For this review, use the dimensioned drawing (mm, ordinates from the lowest corner) and the shaded views. A direction names the side the tool comes from. Coordinates: 2 decimals unless noted, no trailing zeros. Write each loop counter-clockwise with the first axis right and the second up, starting at its lowest first coordinate (ties: lowest second). Pieces come first, ordered by that corner, then holes. Notation, with made-up numbers: M 84,12 L 143,12 A7 ccw 143,25 Z; hole C 72,89.25 d6. An arc over 180 degrees is marked long. Return JSON: item names as keys, results as strings. Group by question number.
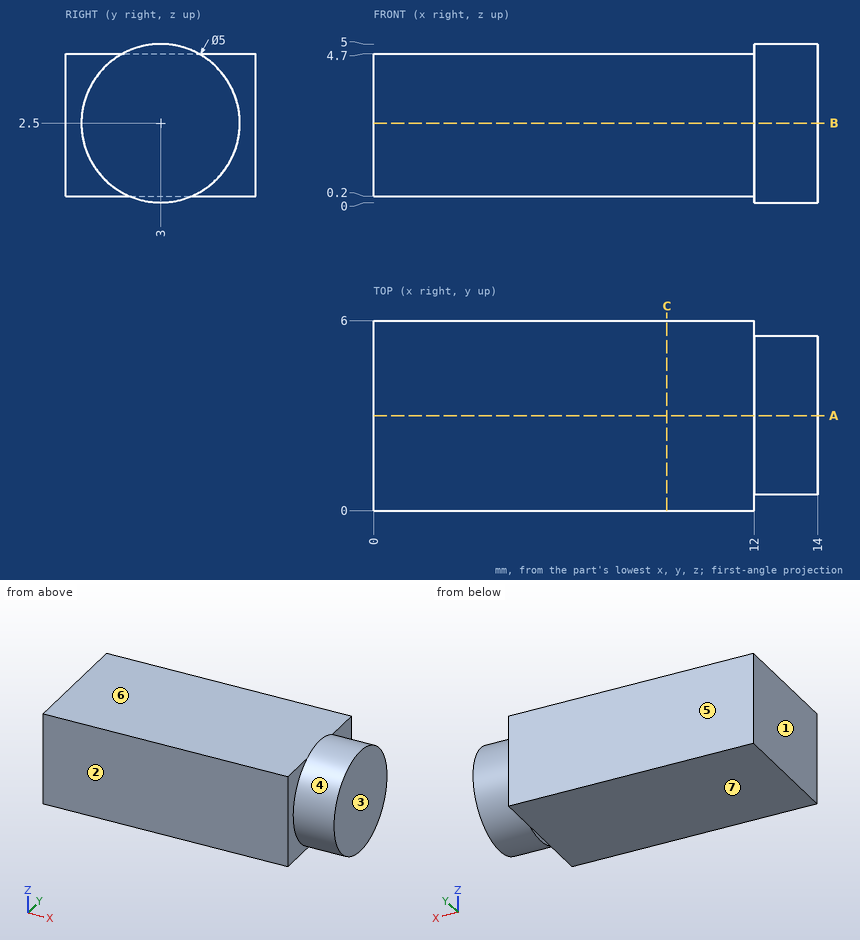
Item 1: Add section B-B (z = 2.5). Write out the cut boundary in (x, y).
Item 2: For line 1 (Z direction, x = 4.5, y = 2.3); line 2 (X direction, y = 5.5, z = 4.3); line 3 (Z direction, x = 13.5, y = 4.2), list the stretches that pass through material, from the lowest coordinate up.
Item 3: Machinability: for the marked faces 4, 5, 6 and 7, which of the approach directions +Z, -Z, +X, -X, +Y, -Y give a long, thin tool a straight path to every point of the face, cutting with its end or side? Answer none if there is none.
Item 4: For pin 1 (3 mm diameter, centred on x = 10, y = 5, fed in from -Z); pin 2 (2 mm diameter, centred on x = 10, y = 1, fed in from +Z), all flat-tipped, find the tip position at first contact; note any pin that passes through.
Item 5: The part is to be moulded in two halves that separate along X. For the marked faces 1, 2 and 3, say which applies: pulls with the +X half, pulls with the -X half, needs draft (parallel to the pull), parting line crosses it, or undercut.
Item 6: Add section A-A (y = 3). Write out the cut boundary in (x, z).
Item 7: Add section C-C (x = 9.25). Write out the cut boundary in (y, z), plus the area to 3 significant figures.
Geometry check:
{
 "1": {"outline": "M 0,0 L 12,0 L 12,0.5 L 14,0.5 L 14,5.5 L 12,5.5 L 12,6 L 0,6 Z"},
 "2": {"line 1": "0.2 to 4.7", "line 2": "0 to 12", "line 3": "0.31 to 4.69"},
 "3": {"face 4": "+X", "face 5": "+Z, -Z, +X, -X, +Y", "face 6": "+Z, -X, +Y, -Y", "face 7": "-Z, -X, +Y, -Y"},
 "4": {"pin 1": "z = 0.2", "pin 2": "z = 4.7"},
 "5": {"face 1": "pulls with the -X half", "face 2": "needs draft", "face 3": "pulls with the +X half"},
 "6": {"outline": "M 0,0.2 L 12,0.2 L 12,0 L 14,0 L 14,5 L 12,5 L 12,4.7 L 0,4.7 Z"},
 "7": {"outline": "M 0,0.2 L 6,0.2 L 6,4.7 L 0,4.7 Z", "area": "27.0 mm^2"}
}
